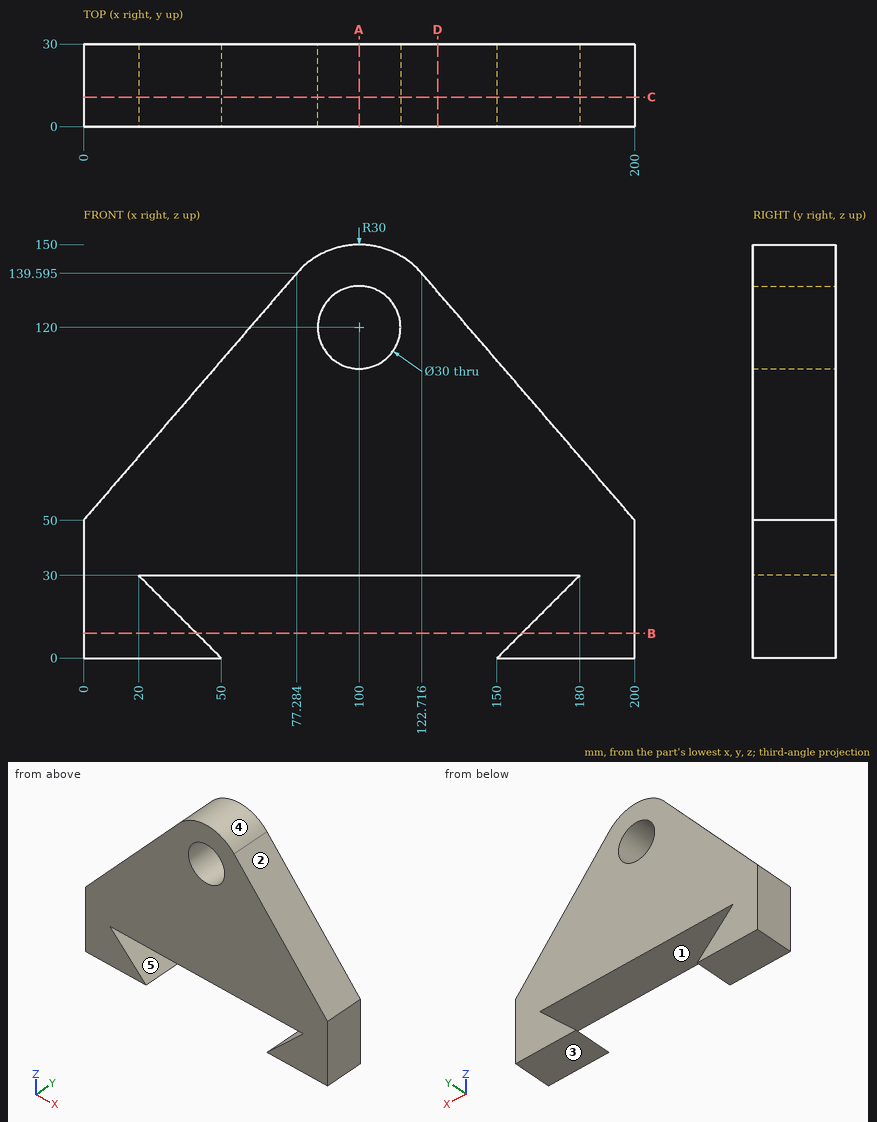
For this review, use the dimensioned drawing (mm, ordinates from the lowest corner) and the shaded views. A direction names the side the tool comes from. Round coordinates to 2 decimals unless told otherwise and drop trailing zeros. Loops run counter-clockwise (first coordinate to the right, second up) from the corner with the lowest first, then second, coordinate; pieces in that order, holes last. Notation, with made-up numbers: M -31.75,89.25 L 3.25,89.25 A17 cw 3.25,110.25 Z; hole C 89,17.25 d7. An arc over 180 degrees is marked long. Answer as a JSON object with one key per item and string values.
(1) Draft analysis for pull direction X (two halves, no side actions). For the marked faces 3, 4 and 5, state which applies: released by +X, released by -X, zero draft, split by the parting line, or undercut.
Resolved:
{"face 3": "zero draft", "face 4": "split by the parting line", "face 5": "undercut"}
(2) Take a section at B-B on z = 9. Give the boundary of the cut face in (x, y).
Resolved:
{"outline": "M 0,0 L 41,0 L 41,30 L 0,30 Z; M 159,0 L 200,0 L 200,30 L 159,30 Z"}
(3) Take a section at D-D on x = 128.5. Give the boundary of the cut face in (y, z).
Resolved:
{"outline": "M 0,30 L 30,30 L 30,132.89 L 0,132.89 Z"}
(4) Take a section at A-A on x = 100. Give the boundary of the cut face in (y, z), and give its area (3 significant figures).
Resolved:
{"outline": "M 0,30 L 30,30 L 30,105 L 0,105 Z; M 0,135 L 30,135 L 30,150 L 0,150 Z", "area": "2,700 mm²"}
(5) Tool access review of the marked faces 1 and 2: name each direction out of +Z, -Z, +X, -X, +Y, -Y from which nothing blocks a thin tool from reaching the whole face with its end or side.
Resolved:
{"face 1": "+Y, -Y", "face 2": "+Z, +X, +Y, -Y"}
(6) Clearance check with flat-ended pins moving along their axes: P1, Ø1.5, axis at y = 17.5, z = 84.5, coming from the +X side; P2, Ø6, axis at y = 15, z = 97.5, coming from the +X side (1 decimal); P3, Ø18, axis at x = 100, z = 120, coming from the -Y side; P4, Ø15, axis at x = 108.5, y = 16, coming from the -Z side. State where each tip first meets the part, or that it passes through.
Resolved:
{"P1": "x = 170.89", "P2": "x = 161.6", "P3": "through", "P4": "z = 30"}
(7) To check wall thickness, follow line 1 along Z through (x, y) = (26.5, 13.5); line 2 along X through (y, z) = (2, 117) (1 decimal); line 3 along Z through (x, y) = (35.5, 10.75) (1 decimal). State the ranges of each line that lie inside material, in increasing order.
Resolved:
{"line 1": "0 to 23.5, 30 to 80.72", "line 2": "57.8 to 85.3, 114.7 to 142.2", "line 3": "0 to 14.5, 30 to 91.2"}
(8) Take a section at C-C on y = 10.75. Give the boundary of the cut face in (x, z) (1 decimal), and give its area (3 significant figures).
Resolved:
{"outline": "M 0,0 L 50,0 L 20,30 L 180,30 L 150,0 L 200,0 L 200,50 L 122.7,139.6 A30 ccw 77.3,139.6 L 0,50 Z; hole C 100,120 d30", "area": "16,700 mm²"}
